from build123d import *

# Parameters (mm, degrees)
F0_R     = 8
F1_DEPTH = 20
F2_W     = 19
F2_H     = 4
F3_DEPTH = 8
F4_R     = 1
F5_DEPTH = 8
F6_R     = 2


with BuildPart() as f1:
    # F0 (on Top) → F1 (new body)
    with BuildSketch(Plane.XY):
        Circle(F0_R)
    extrude(amount=F1_DEPTH)

    # F2 (on face) → F3 (cut)
    with BuildSketch(Plane(origin=(0, 0, 0), x_dir=(1, 0, 0), z_dir=(0, 0, -1))):
        Rectangle(F2_W, F2_H)
    extrude(amount=-F3_DEPTH, mode=Mode.SUBTRACT)

    # F4 (on Front) → F5 (cut, symmetric)
    with BuildSketch(Plane.XZ):
        with Locations((0, 3)):
            Circle(F4_R)
    extrude(amount=F5_DEPTH, both=True, mode=Mode.SUBTRACT)

    # F6
    f6_edges = [f1.edges().sort_by_distance(p)[0] for p in [
        (0, -2, 0),
        (0, 2, 0),
    ]]
    fillet(f6_edges, radius=F6_R)


solid = f1.part
Check sheet for the modelled part. Datum: model origin and axes. Units: mm. A direction names the side the tool comes from. Give positions to 0.01 mm unless a question says otherwise; leave off trailing zeros. Write each loop counter-clockwise with the first axis right and the second up, starting at its lowest first coordinate (ties: lowest second). Pieces come first, ordered by that corner, then holes. Notation, with made-up numbers: (38.5, 47) -> (83.5, 47) arc R29 ccw to (83.5, 67) -> close; hole circle Ø9 at (48, 22). An arc over 180 degrees is marked (long way). Write item = value, one per line.
Item 1: Scan lines: probe 1 along Z at (x, y) = (0, 4.5); probe 2 along X at (y, z) = (4, 3); probe 3 along X at (y, z) = (-6.25, 3). Record each from-to range of solid material in increasing order. Write a range as from..to.
Output:
probe_1 = 0..2, 4..20
probe_2 = -6.93..-1, 1..6.93
probe_3 = -4.99..-1, 1..4.99
Item 2: Sectioned sample at B-B on y = -6.5. Record the boundary of the cut face in (x, z).
Output:
outline = (-4.66, 0) -> (4.66, 0) -> (4.66, 20) -> (-4.66, 20) -> close; hole circle Ø2 at (0, 3)
Item 3: Tool access check on faces 1 (the cylindrical face through (0.11, -2.6, 0.57)), 2 (the flat face through (0, 6, 0)). Record the directions out of +Z, -Z, +X, -X, +Y, -Y that give a thin tool (end or side, any length) a straight path to the whole face; none if there is none.
Output:
face_1 = -Z, +X, -X
face_2 = -Z, +X, -X, +Y, -Y
Item 4: Sectioned sample at A-A on z = 3. Record the boundary of the cut face in (x, y).
Output:
outline = (-7.75, -2) arc R8 ccw to (-1, -7.94) -> (-1, -2) -> close; (-7.75, 2) -> (-1, 2) -> (-1, 7.94) arc R8 ccw to start; (1, -7.94) arc R8 ccw to (7.75, -2) -> (1, -2) -> close; (1, 2) -> (7.75, 2) arc R8 ccw to (1, 7.94) -> close
Item 5: Release check for a two-part mould opening along Y. For faces 3 (the flat face through (0, 2, 5)), 4 (the cylindrical face through (7.39, -3.06, 9.86)), 5 (the flat face through (0, -6, 0)) record: +Y half, -Y half, draft (parallel to the pull), parting line (faces both ways), or undercut.
Output:
face_3 = undercut
face_4 = parting line
face_5 = draft
Item 6: Gauge pin test, flat ends, axial feed: pin 1 (1.8 mm diameter, centred on x = 1.5, z = 5.5, fed in from +Y); pin 2 (5 mm diameter, centred on y = 6, z = 2, fed in from +X); pin 3 (1.2 mm diameter, centred on x = 0, z = 3, fed in from +Y); pin 4 (2 mm diameter, centred on y = -6, z = 5, fed in from -X) (3 decimals). Record the tip position at first contact, or that the pin passes through.
Output:
pin_1 = 7.98
pin_2 = 7.19
pin_3 = through
pin_4 = -6.245
Item 7: Sectioned sample at C-C on x = -1.5. Record the boundary of the cut face in (y, z), and give its area (3 significant figures).
Output:
outline = (-7.86, 0) -> (-4, 0) arc R2 ccw to (-2, 2) -> (-2, 8) -> (2, 8) -> (2, 2) arc R2 ccw to (4, 0) -> (7.86, 0) -> (7.86, 20) -> (-7.86, 20) -> close
area = 281 mm^2
Item 8: Sectioned sample at D-D on y = 0. Record the boundary of the cut face in (x, z).
Output:
outline = (-8, 8) -> (8, 8) -> (8, 20) -> (-8, 20) -> close
